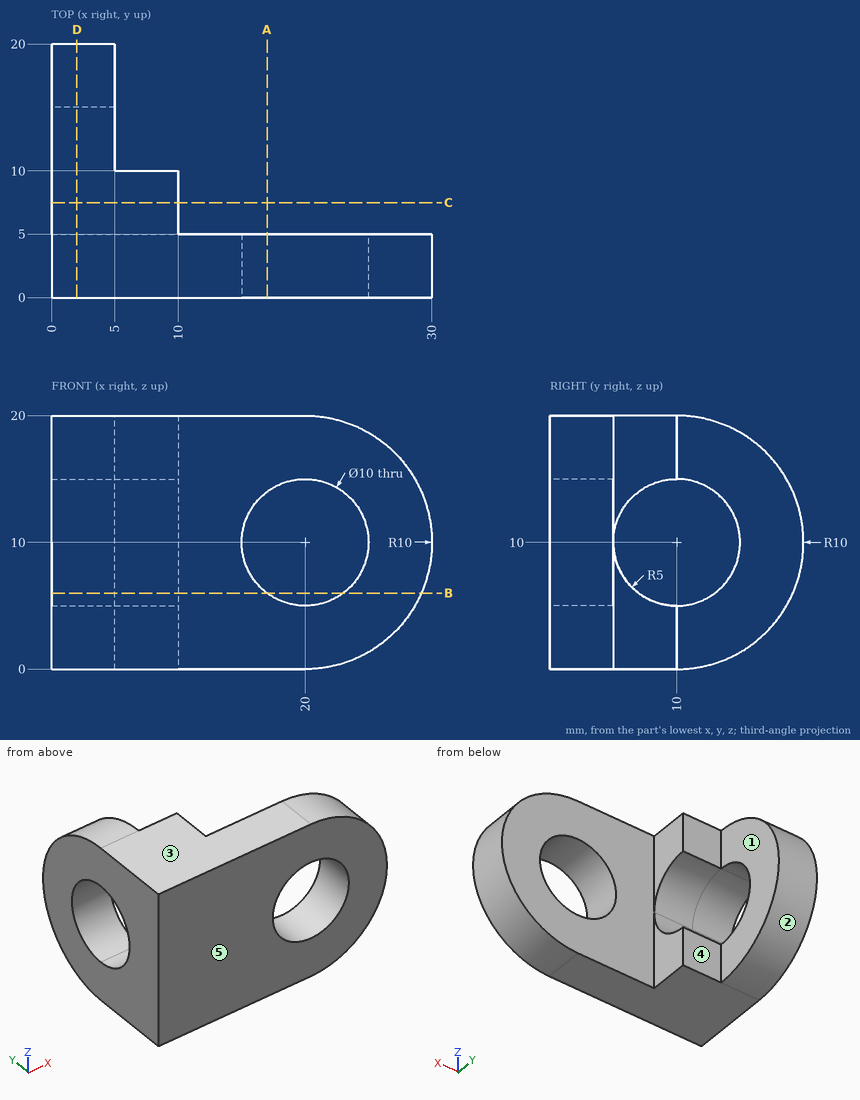
Input: dimensioned drawing with shaded views. Units: mm. Origin: part minimum x, y, z. A direction names the side the tool comes from. Give positions to 0.01 mm unless a question says otherwise; leave off trailing zeros. Order: outer loops, then holes, each group sorted by start corner. A loop starts at its lowest first (then second) coordinate and runs counter-clockwise, first axis right, second up. Notation, with made-up numbers: (48, 39.5) -> (70, 39.5) arc R28 ccw to (70, 60.5) -> close; hole circle Ø3 at (4.25, -36.75). An arc over 180 degrees is marked (long way). Use one line per item in the form item = value.
1) Section C-C, the plane y = 7.5. Return loops of the section in (x, z), and give its area (3 significant figures).
Response values:
outline = (0, 0) -> (10, 0) -> (10, 5.67) -> (0, 5.67) -> close; (0, 14.33) -> (10, 14.33) -> (10, 20) -> (0, 20) -> close
area = 113 mm^2
2) Section B-B, the plane z = 6. Return loops of the section in (x, y).
Response values:
outline = (0, 0) -> (17, 0) -> (17, 5) -> (10, 5) -> (10, 7) -> (0, 7) -> close; (0, 13) -> (5, 13) -> (5, 19.17) -> (0, 19.17) -> close; (23, 0) -> (29.17, 0) -> (29.17, 5) -> (23, 5) -> close
3) Reachability of the marked faces 1 and 2 from +Z, -Z, +X, -X, +Y, -Y: full face, straight path, thin tool, end or side. Return the list, or none.
Response values:
face_1 = +Z, -Z, +X, +Y
face_2 = +X, -X, +Y
4) Section D-D, the plane x = 2. Return loops of the section in (y, z).
Response values:
outline = (0, 0) -> (10, 0) arc R10 ccw to (10, 20) -> (0, 20) -> close; hole circle Ø10 at (10, 10)
5) Mould query, pull axis Y, two halves, no side actions, for the marked faces 3, 4 and 5. Classes: pulls with the +Y half, pulls with the -Y half, needs draft (parallel to the pull), parting line crosses it, or undercut.
Response values:
face_3 = needs draft
face_4 = pulls with the +Y half
face_5 = pulls with the -Y half
6) Line query: probe 1 along X at (y, z) = (1.9, 10); probe 2 along Z at (x, y) = (20, 3.95); probe 3 along Y at (x, z) = (20.75, 4.75). Output: solid intervals per line, ascending.
Response values:
probe_1 = 0 to 15, 25 to 30
probe_2 = 0 to 5, 15 to 20
probe_3 = 0 to 5
7) Section A-A, the plane x = 17. Return loops of the section in (y, z).
Response values:
outline = (0, 0) -> (5, 0) -> (5, 6) -> (0, 6) -> close; (0, 14) -> (5, 14) -> (5, 20) -> (0, 20) -> close
8) First-contact query: pin 1 Ø8 at (y, z) = (15.5, 11) entering from +X; pin 2 Ø10 at (x, y) = (7, 5) entering from -Z; pin 3 Ø6 at (x, z) = (22, 6) entering from +Y; pin 4 Ø1.5 at (x, z) = (8.5, 2.5) entering from +Y. Flat tips, straight axial feed; report the tip coordinate or a pass-through.
Response values:
pin_1 = 5
pin_2 = 0
pin_3 = 5
pin_4 = 10
